Build history of the part. All positions in model axes, mm. Face numbers are marked on the shaded views. A direction names the side the tool comes from. Round coordinates to 2 decimals unless told otherwise and drop trailing zeros. Order: outer loops, then holes, each group sorted by start corner. A loop starts at its lowest first (then second) coordinate and runs counter-clockwise, first axis right, second up. Notation, with made-up numbers: M 85.25,-26 L 94.25,-26 A6 cw 94.25,-17 Z; hole C 48,0 d4. An arc over 180 degrees is marked long. One line per item, written item: value. Start each with the question number.
Item 1: Band-saw the part on D-D, the plane z = 20.5. Write the cut outline in (x, y), then the cut area to 3 significant figures.
Item 2: Tool access for the marked faces 4, 5 and 6: list every direction of +Z, -Z, +X, -X, +Y, -Y with a clear straight run to the whole face (end or side of a thin tool).
Item 3: Two-plate mould, pull along Y, no slides. Class the marked faces 1, 2 and 3: +Y half, -Y half, draft (parallel to the pull), parting line (faces both ways), or undercut.
Item 4: Probe L1, parallel to Y at x = 0, z = 80.5; L2, parallel to Z at x = -22, y = 72; L3, parallel to X at y = -52.5, z = 13.5. List the from-to ranges inside material, lowest first.
Item 5: Band-saw the part on B-B, the plane y = -47.5. Write the cut outline in (x, z).
Item 6: Band-saw the part on C-C, the plane x = -4.5. Write the cut outline in (y, z), then the cut area to 3 significant figures.
Item 7: Pin check, flat tips, straight feed: pin 1 (21 mm diameter, centred on x = -26, y = -71, fed in from -Z); pin 2 (20.5 mm diameter, centred on x = 27.5, y = -32.5, fed in from +Z); pin 3 (1.5 mm diameter, centred on y = -10.5, z = 72.5, fed in from +X). Stop position of each tip, or through.
Item 8: Band-saw the part on A-A, the plane z = 85. Write the cut outline in (x, y).
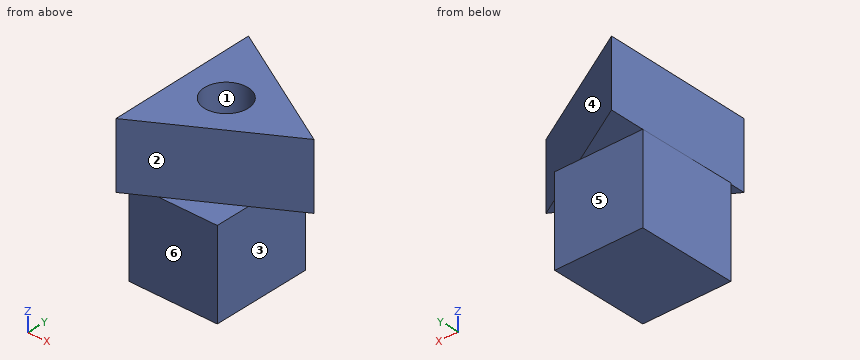
```python
from build123d import *

# Parameters (mm, degrees)
F0_W     = 102.221594
F0_H     = 114.750422
F1_DEPTH = 101.6
F3_DEPTH = 76.2
F4_R     = 25.169937
F5_DEPTH = 147.32


with BuildPart() as f1:
    # F0 (on Top) → F1 (new body)
    with BuildSketch(Plane.XY):
        Rectangle(F0_W, F0_H)
    extrude(amount=F1_DEPTH)

    # F2 (on face) → F3 (join)
    with BuildSketch(Plane.XY.offset(101.6)):
        Polygon((-49.475546, -76.307332), (100.875381, 12.719793), (-51.399834, 98.413953), align=None)
    extrude(amount=F3_DEPTH)

    # F4 (on face) → F5 (cut)
    with BuildSketch(Plane.XY.offset(177.8)):
        with Locations((0, 11.758941)):
            Circle(F4_R)
    extrude(amount=-F5_DEPTH, mode=Mode.SUBTRACT)


solid = f1.part
```
Output:
1. outline: M -51.11,-57.38 L 51.11,-57.38 L 51.11,57.38 L -51.11,57.38 Z
1. area: 11,700 mm²
2. face 4: +Z, +X, +Y
2. face 5: -Z, +X, -X, +Y
2. face 6: -Z, +X, -X, -Y
3. face 1: undercut
3. face 2: -Y half
3. face 3: draft
4. L1: y = -57.38 to -13.41, 36.93 to 57.38
4. L2: z = 101.6 to 177.8
4. L3: x = -51.11 to 51.11
5. outline: M -51.11,0 L 51.11,0 L 51.11,101.6 L -0.83,101.6 L -0.83,177.8 L -49.79,177.8 L -49.79,101.6 L -51.11,101.6 Z
6. outline: M -57.38,0 L 57.38,0 L 57.38,101.6 L 72.02,101.6 L 72.02,177.8 L 36.52,177.8 L 36.52,30.48 L -13.01,30.48 L -13.01,177.8 L -49.68,177.8 L -49.68,101.6 L -57.38,101.6 Z
6. area: 13,600 mm²
7. pin 1: stops at z = 101.6
7. pin 2: stops at z = 177.8
7. pin 3: stops at x = 51.11
8. outline: M -51.11,-57.38 L 51.11,-57.38 L 51.11,57.38 L -51.11,57.38 Z; hole C 0,11.76 d50.34
